from build123d import *

# Parameters (mm, degrees)
F0_R     = 1.5
F0_W     = 6.9863945246
F0_H     = 1.5458728885
F1_DEPTH = 1
F2_DEPTH = 25
F3_W     = 12.2058418553
F3_H     = 2
F4_DEPTH = 25
F6_DEPTH = 0.5
F7_DEPTH = 25
F8_DEPTH = 25


with BuildPart() as f1:
    # F0 (on Right) → F1 (new body)
    with BuildSketch(Plane.YZ):
        with BuildLine():
            Line((-7.5285646403, -1.7005902689), (7.5285646403, -1.7005902689))
            ThreePointArc((7.5285646403, -1.7005902689), (10.8904195418, -2.8648129153), (13, 0))
            Line((13, 0), (13, 3.5))
            Line((13, 3.5), (-13, 3.5))
            Line((-13, 3.5), (-13, 0))
            ThreePointArc((-13, 0), (-10.8904195418, -2.8648129153), (-7.5285646403, -1.7005902689))
        make_face()
        with Locations((-10, 0)):
            Circle(F0_R, mode=Mode.SUBTRACT)
        with Locations((10, 0)):
            Circle(F0_R, mode=Mode.SUBTRACT)
        Polygon((6.9863945246, 0), (0, 0), (-6.9863945246, 0), (-6.9863945246, 1.5458728885), (0, 1.5458728885), (6.9863945246, 1.5458728885), align=None, mode=Mode.SUBTRACT)
        with Locations((3.4931972623, 0.7729364443)):
            Rectangle(F0_W, F0_H)
    extrude(amount=F1_DEPTH)

    # F0 (on Right) → F2 (join)
    with BuildSketch(Plane.YZ):
        with Locations((3.4931972623, 0.7729364443)):
            Rectangle(F0_W, F0_H)
    extrude(amount=F2_DEPTH)

    # F3 (on face) → F4 (cut)
    with BuildSketch(Plane(origin=(0, 0, 0), x_dir=(1, 0, 0), z_dir=(0, 0, -1))):
        with Locations((16.3970790723, -3.5)):
            Rectangle(F3_W, F3_H)
    extrude(amount=-F4_DEPTH, mode=Mode.SUBTRACT)

    # F5 (on face) → F6 (join, symmetric)
    with BuildSketch(Plane.XZ):
        with BuildLine():
            ThreePointArc((0, -5.004207138), (4.7964248116, -3.6540201663), (8.1841722131, 0))
            Line((8.1841722131, 0), (0, 0))
            Line((0, 0), (0, -5.004207138))
        make_face()
        with BuildLine():
            Line((0, 0), (8.1841722131, 0))
            ThreePointArc((8.1841722131, 0), (4.5027216519, 2.7135344455), (0, 3.5146868322))
            Line((0, 3.5146868322), (0, 0))
        make_face()
    extrude(amount=F6_DEPTH, both=True)

    # F0 (on Right) → F7 (join)
    with BuildSketch(Plane.YZ):
        with Locations((-3.4931972623, 0.7729364443)):
            Rectangle(F0_W, F0_H)
    extrude(amount=F7_DEPTH)

    # F3 (on face) → F8 (cut)
    with BuildSketch(Plane(origin=(0, 0, 0), x_dir=(1, 0, 0), z_dir=(0, 0, -1))):
        with Locations((16.3970790723, 3.5)):
            Rectangle(F3_W, F3_H)
    extrude(amount=-F8_DEPTH, mode=Mode.SUBTRACT)


solid = f1.part
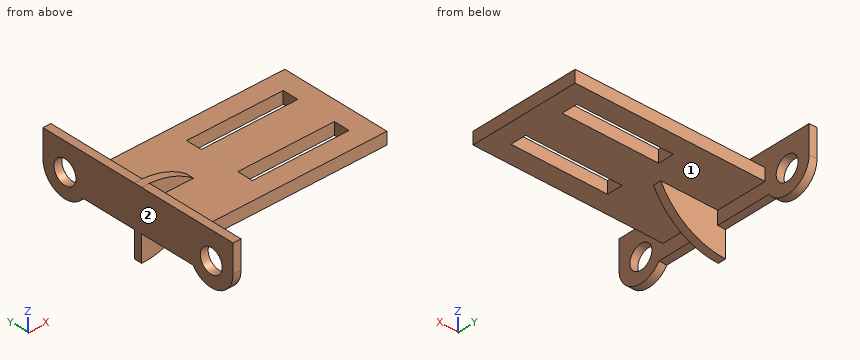
Work out the finished part from the listing and answer in its coordinate system (mm). Face numbers are marked on the shaded views. A direction names the side the tool comes from. Give positions to 0.01 mm unless a question says otherwise; leave off trailing zeros. Order: outer loops, then holes, each group sorted by start corner. A loop starts at its lowest first (then second) coordinate and runs counter-clockwise, first axis right, second up. Notation, with made-up numbers: M 36.5,75.25 L 58.5,75.25 A10 ccw 58.5,88.25 Z; hole C 2.25,-12 d2. An arc over 180 degrees is marked long. Return JSON: item names as keys, results as strings.
Q1. Find section B-B, the plane x = 11. Write down the section's boundary in (y, z), and give its area (3 significant figures).
Answer below:
{"outline": "M -6.99,0 L -4.5,0 L -4.5,1.55 L -6.99,1.55 Z; M -2.5,0 L 2.5,0 L 2.5,1.55 L -2.5,1.55 Z; M 4.5,0 L 6.99,0 L 6.99,1.55 L 4.5,1.55 Z", "area": "15.4 mm^2"}
Q2. Find section A-A, the plane y = -10. Write down the section's boundary in (x, z).
Answer below:
{"outline": "M 0,-3 L 1,-3 L 1,-1.5 L 0,-1.5 Z; M 0,1.5 L 1,1.5 L 1,3.5 L 0,3.5 Z"}
Q3. Each of these flat-tipped pins is pushed along its axis until it touches: pin 1 (1.6 mm diameter, centred on x = 5, z = 3, fed in from -Y); pin 2 (1.5 mm diameter, centred on x = 14.5, z = -2.5, fed in from -Y); pin 3 (12 mm diameter, centred on x = 21.5, y = 8.5, fed in from +Z); pin 4 (6 mm diameter, centred on x = 5, y = -8, fed in from -Z). Where does it stop, or does it pass through?
Answer below:
{"pin 1": "stops at y = -0.5", "pin 2": "passes through", "pin 3": "stops at z = 1.55", "pin 4": "stops at z = 0"}
Q4. Find section D-D, the plane x = 3.25. Write down the section's boundary in (y, z), and give its area (3 significant figures).
Answer below:
{"outline": "M -6.99,0 L -0.5,0 L -0.5,-4.41 L 0.5,-4.41 L 0.5,0 L 6.99,0 L 6.99,1.55 L 0.5,1.55 L 0.5,3.16 L -0.5,3.16 L -0.5,1.55 L -6.99,1.55 Z", "area": "27.6 mm^2"}
Q5. Find section C-C, the plane y = -5. Write down the section's boundary in (x, z), and give its area (3 significant figures).
Answer below:
{"outline": "M 0,-1.7 L 1,-1.7 L 1,0 L 25,0 L 25,1.55 L 1,1.55 L 1,3.5 L 0,3.5 Z", "area": "42.3 mm^2"}
Q6. Which of the six approach directions +Z, -Z, +X, -X, +Y, -Y give full straight-line access (tool end or side, diameter ignored) to the marked faces 1 and 2?
Answer below:
{"face 1": "-Z, +X", "face 2": "+Z, -Z, -X, +Y, -Y"}
Q7. Find the intervals of material crossed by line 1 along Y through (x, z) = (15.25, 1.25); line 2 along Z through (x, y) = (0.7, -10); line 3 along X through (y, z) = (-7.75, 2.5), in increasing order. Write a range as [from, to].
Answer below:
{"line 1": "y = [-6.99, -4.5], [-2.5, 2.5], [4.5, 6.99]", "line 2": "z = [-3, -1.5], [1.5, 3.5]", "line 3": "x = [0, 1]"}
